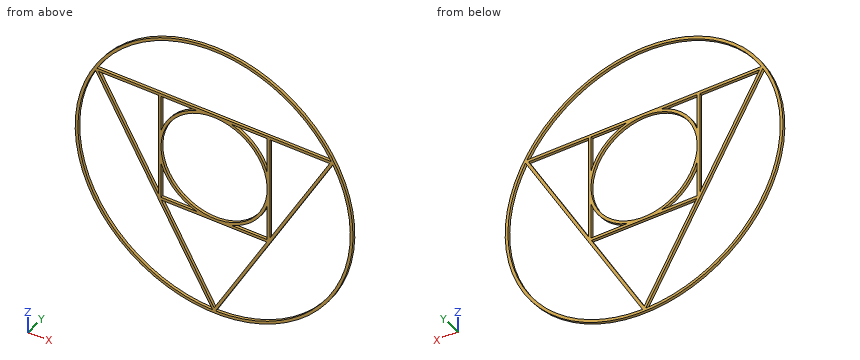
from build123d import *

# Parameters (mm, degrees)
SKETCH1_R           = 182.705
SKETCH1_R_2         = 69.823485805
BOSS_EXTRUDE4_DEPTH = 3.61


with BuildPart() as part:
    # Sketch1 → Boss-Extrude4 (new body)
    with BuildSketch(Plane(origin=(0, 0, 0), x_dir=(1, 0, 0), z_dir=(0, 1, 0))):
        with Locations(Location((0, 0, 0), (0, 0, 270))):
            Circle(SKETCH1_R)
        Polygon((-73.433485805, -87.7425), (-151.974467983, -87.7425), (-73.433485805, 48.294471609), align=None, mode=Mode.SUBTRACT)
        with BuildLine():
            Line((-22.741100842, -87.7425), (-69.823485805, -87.7425))
            Line((-69.823485805, -87.7425), (-69.823485805, -40.660115037))
            ThreePointArc((-69.823485805, -40.660115037), (-51.925315779, -69.844329974), (-22.741100842, -87.7425))
        make_face(mode=Mode.SUBTRACT)
        with Locations(Location((0, -17.919014195, 0), (0, 0, 270))):
            Circle(SKETCH1_R_2, mode=Mode.SUBTRACT)
        with BuildLine():
            ThreePointArc((154.04460318, -91.3525), (0, -179.095), (-154.04460318, -91.3525))
            Line((-154.04460318, -91.3525), (-73.433485805, -91.3525))
            Line((-73.433485805, -91.3525), (73.433485805, -91.3525))
            Line((73.433485805, -91.3525), (154.04460318, -91.3525))
        make_face(mode=Mode.SUBTRACT)
        with BuildLine():
            Line((69.823485805, -40.660115037), (69.823485805, -87.7425))
            Line((69.823485805, -87.7425), (22.741100842, -87.7425))
            ThreePointArc((22.741100842, -87.7425), (51.925315779, -69.844329974), (69.823485805, -40.660115037))
        make_face(mode=Mode.SUBTRACT)
        Polygon((151.974467983, -87.7425), (73.433485805, -87.7425), (73.433485805, 48.294471609), align=None, mode=Mode.SUBTRACT)
        with BuildLine():
            Line((-69.823485805, 51.904471609), (-22.741100842, 51.904471609))
            ThreePointArc((-22.741100842, 51.904471609), (-51.925315779, 34.006301583), (-69.823485805, 4.822086647))
            Line((-69.823485805, 4.822086647), (-69.823485805, 51.904471609))
        make_face(mode=Mode.SUBTRACT)
        with BuildLine():
            ThreePointArc((-156.135887289, -87.730289669), (-155.100819691, 89.5475), (-2.091284109, 179.082789669))
            Line((-2.091284109, 179.082789669), (-156.135887289, -87.730289669))
        make_face(mode=Mode.SUBTRACT)
        Polygon((-69.265016861, 55.514471609), (0, 175.485), (69.265016861, 55.514471609), align=None, mode=Mode.SUBTRACT)
        with BuildLine():
            Line((22.741100842, 51.904471609), (69.823485805, 51.904471609))
            Line((69.823485805, 51.904471609), (69.823485805, 4.822086647))
            ThreePointArc((69.823485805, 4.822086647), (51.925315779, 34.006301583), (22.741100842, 51.904471609))
        make_face(mode=Mode.SUBTRACT)
        with BuildLine():
            ThreePointArc((2.091284109, 179.082789669), (155.100819691, 89.5475), (156.135887289, -87.730289669))
            Line((156.135887289, -87.730289669), (2.091284109, 179.082789669))
        make_face(mode=Mode.SUBTRACT)
    extrude(amount=BOSS_EXTRUDE4_DEPTH)


solid = part.part
Source: CAD feature listing. Evaluate the final solid. Frame: model axes, mm. Coordinates: 2 decimals unless noted, no trailing zeros. Loops run counter-clockwise (first coordinate to the right, second up) from the corner with the lowest first, then second, coordinate; pieces in that order, holes last. Notation, with made-up numbers: M 64.5,57 L 102.5,57 A26 cw 102.5,96 Z; hole C -17,68 d3. An arc over 180 degrees is marked long. Answer in a Markdown table with one row per item.
Q1. Section B-B on x = -116.5. Return the cut outline in (y, z).
Answers below:
| item | result |
|---|---|
| outline | M 0,-140.74 L 3.61,-140.74 L 3.61,-136.02 L 0,-136.02 Z; M 0,19.08 L 3.61,19.08 L 3.61,26.3 L 0,26.3 Z; M 0,87.74 L 3.61,87.74 L 3.61,91.35 L 0,91.35 Z; M 0,136.02 L 3.61,136.02 L 3.61,140.74 L 0,140.74 Z |
Q2. First-contact query: pin 1 (1.1 mm diameter, centred on x = -118, y = 1.5, fed in from -Z); pin 2 (5 mm diameter, centred on x = -42, z = -41, fed in from -Y); pin 3 (1.8 mm diameter, centred on x = 118, y = 1.5, fed in from -Z); pin 4 (1.8 mm diameter, centred on x = 40, y = 1.5, fed in from +Z). Flat tips, straight axial feed; report the tip coordinate or a pass-through.
Answers below:
| item | result |
|---|---|
| pin 1 | stops at z = -139.95 |
| pin 2 | stops at y = 0 |
| pin 3 | stops at z = -140.25 |
| pin 4 | stops at z = 178.47 |
Q3. Section D-D on z = -120. Return the cut outline in (x, y), plus the area to 3 significant figures.
Answers below:
| item | result |
|---|---|
| outline | M -137.77,0 L -132.95,0 L -132.95,3.61 L -137.77,3.61 Z; M -36.2,0 L -32.03,0 L -32.03,3.61 L -36.2,3.61 Z; M 32.03,0 L 36.2,0 L 36.2,3.61 L 32.03,3.61 Z; M 132.95,0 L 137.77,0 L 137.77,3.61 L 132.95,3.61 Z |
| area | 64.9 mm^2 |
Q4. Ray query, probe 1 along Z at (x, y) = (-94, 2.55); probe 2 along X at (y, z) = (0.7, 18); probe 3 along X at (y, z) = (0.6, -142.5). Return the intervals inside material, ascending. Write a range as from..to.
Answers below:
| item | result |
|---|---|
| probe 1 | z = -156.67..-152.44, -19.89..-12.67, 87.74..91.35, 152.44..156.67 |
| probe 2 | x = -181.82..-178.19, -115.88..-111.71, -73.43..-69.82, 69.82..73.43, 111.71..115.88, 178.19..181.82 |
| probe 3 | x = -114.35..-108.48, -23.21..-19.04, 19.04..23.21, 108.48..114.35 |
Q5. Section A-A on z = -16. State how many separate pieces and enclosed holes the cut face has, plus the area to 3 significant figures.
Answers below:
| item | result |
|---|---|
| separate pieces | 8 |
| enclosed holes | 0 |
| area | 112 mm^2 |
